Verification items for this drawing (mm, ordinates from the low corner). A direction names the side the tool comes from. Give positions to 0.01 mm unless a question says otherwise; leave off trailing zeros. Loops run counter-clockwise (first coordinate to the right, second up) from the corner with the lowest first, then second, coordinate; pieces in that order, holes last. Notation, with made-up numbers: (-26.5, 60) - (-1.5, 60) arc R6 ccw to (-1.5, 70) - close; hole circle Ø1 at (5, 53.25). An arc over 180 degrees is marked (long way). One line per question, with ' | ' between items. Start each with the question number.
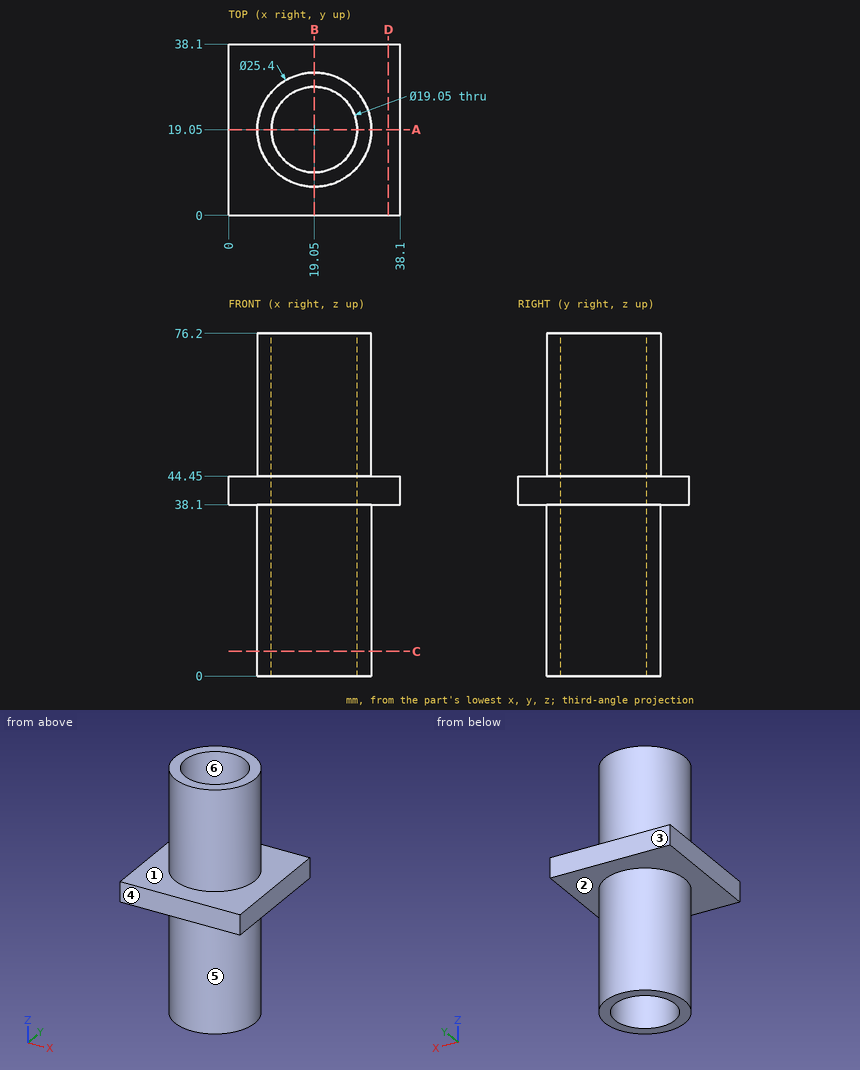
(1) Section check A-A, the plane y = 19.05. Record the boundary of the cut face in (x, z) (3 decimals), and give its area (3 significant figures).
(2) Section check C-C, the plane z = 5.5. Record the boundary of the cut face in (x, y) (3 decimals), and give its area (3 significant figures).
(3) Mould release check, pull along X, two halves, no side actions. Record for the marked faces 4, 5 and 6: pulls with the +X half, pulls with the -X half, needs draft (parallel to the pull), parting line crosses it, or undercut.
(4) Section check D-D, the plane x = 35.5. Record the boundary of the cut face in (y, z).
(5) Depth check by flat-ended pin: pin 1 Ø3 at (x, z) = (13, 30.5) entering from +Y; pin 2 Ø5 at (y, z) = (5, 17) entering from +X; pin 3 Ø4 at (x, z) = (31, 21.5) entering from +Y. Enter the tip coordinate at first touch or a pass-through.
(6) Material ranges on line 1 (Y direction, x = 19.05, z = 55.5) (3 decimals); line 2 (X direction, y = 19, z = 46); line 3 (Z direction, x = 14, y = 7), recorded low to high.
(7) Tool access check on the marked faces 1, 2 and 3. Record the directions out of +Z, -Z, +X, -X, +Y, -Y that give a thin tool (end or side, any length) a straight path to the whole face; none if there is none.
Numbers:
1) outline: (0, 38.1) - (6.35, 38.1) - (6.35, 0) - (9.525, 0) - (9.525, 76.2) - (6.35, 76.2) - (6.35, 44.45) - (0, 44.45) - close; (28.575, 0) - (31.75, 0) - (31.75, 38.1) - (38.1, 38.1) - (38.1, 44.45) - (31.75, 44.45) - (31.75, 76.2) - (28.575, 76.2) - close | area: 565 mm^2
2) outline: circle Ø25.4 at (19.05, 19.05); hole circle Ø19.05 at (19.05, 19.05) | area: 222 mm^2
3) face 4: needs draft | face 5: parting line crosses it | face 6: undercut
4) outline: (0, 38.1) - (38.1, 38.1) - (38.1, 44.45) - (0, 44.45) - close
5) pin 1: y = 30.91 | pin 2: x = 24.33 | pin 3: y = 26.94
6) line 1: 6.35 to 9.525, 28.575 to 31.75 | line 2: 6.35 to 9.53, 28.57 to 31.75 | line 3: 38.1 to 44.45
7) face 1: +Z | face 2: -Z | face 3: +Z, -Z, +X, -X, +Y
